Autodesk Inventor part; units mm, degrees
ref_plane "YZ Plane" through (0, 0, 0) normal (1, 0, 0) x (0, 1, 0)
ref_plane "XZ Plane" through (0, 0, 0) normal (0, 1, 0) x (-1, 0, 0)
ref_plane "XY Plane" through (0, 0, 0) normal (0, 0, 1) x (1, 0, 0)
sketch "Skizze1" plane through (0, 0, 0) normal (0, 0, 1) x (1, 0, 0)
  line L0 (13.8, 20) -> (-13.8, 20)
  line L1 (-13.8, 20) -> (-13.8, -20)
  line L2 (-13.8, -20) -> (13.8, -20)
  line L3 (13.8, 20) -> (-13.8, -20) construction
  line L4 (-13.8, 20) -> (13.8, -20) construction
  line L5 (13.8, 20) -> (13.8, 6.65) construction
  line L6 (13.8, 6.65) -> (10.7, 6.65)
  line L7 (-13.8, 0) -> (-0.95, 0) construction
  arc A0 (4.1513, 4.266) -> (4.1513, -4.266) centre (-0.95, 0) ccw
  line L8 (13.8, 6.65) -> (13.8, -6.65) construction
  line L9 (13.8, -6.65) -> (10.7, -6.65)
  line L10 (13.8, -20) -> (13.8, -6.65)
  line L11 (13.8, 6.65) -> (13.8, 20)
  line L12 (10.7, 6.65) -> (4.1513, 4.266)
  line L13 (10.7, -6.65) -> (4.1513, -4.266)
  point P0 (0, 0)
  dimension "d0" = 27.6
  dimension "d1" = 40
  dimension "d2" = 13.35
  dimension "d3" = 3.1
  dimension "d4" = 12.85
  dimension "d5" = 13.3
  dimension "d7" = 13.3
  dimension "d8" = 3.1
  dimension "d24" = 6.5487
  dimension "d25" = 6.5487
extrude "Extrusion1" add sketch "Skizze1" along normal blind 39
sketch "Skizze2" plane through (-13.8, -20, 0) normal (-1, 0, 0) x (0, 0, 1)
  line L0 (0, 40) -> (39, 40) construction
  line L1 (0, 0) -> (39, 0) construction
  line L2 (0, 40) -> (39, 0) construction
  line L3 (39, 40) -> (0, 0) construction
  line L4 (6.5, 6) -> (32.5, 6) construction
  line L5 (32.5, 6) -> (32.5, 34) construction
  line L6 (32.5, 34) -> (6.5, 34) construction
  line L7 (6.5, 34) -> (6.5, 6) construction
  line L8 (6.5, 6) -> (32.5, 34) construction
  line L9 (32.5, 6) -> (6.5, 34) construction
  point P0 (0, 20)
  point P1 (19.5, 20)
  dimension "d12" = 26
  dimension "d13" = 28
hole "Bohrung1" at (-13.8, 14, 6.5) at (-13.8, 14, 32.5) at (-13.8, -14, 32.5) at (-13.8, -14, 6.5) direction (1, 0, 0) diameter 3.242 depth 11.8 tip angle 118
chamfer "Fase1" distance 0.5 angle 45 26 edges at (13.8, 13.325, 39) (13.8, 13.325, 0) (13.8, -13.325, 0) (13.8, -13.325, 39) (13.8, -20, 19.5) (0, -20, 39) (-13.8, 0, 39) (0, 20, 39) (-13.8, 20, 19.5) (0, 20, 0) (13.8, 6.65, 19.5) (13.8, -6.65, 19.5) (-7.6, 0, 39) (7.4257, -5.458, 39) (12.25, -6.65, 39) (7.4257, 5.458, 39) (12.25, 6.65, 39) (-7.6, 0, 0) (7.4257, -5.458, 0) (12.25, -6.65, 0) (12.25, 6.65, 0) (7.4257, 5.458, 0) (0, -20, 0) (-13.8, -20, 19.5) (-13.8, 0, 0) (13.8, 20, 19.5)
chamfer_without_effect "Fase2"
properties part number "Führungswagen" material "Aluminium 6061"
CAD build for the part. Positions are in the model's coordinates, mm. A direction names the side the tool comes from. Coordinates: 2 decimals unless noted, no trailing zeros. Loops run counter-clockwise (first coordinate to the right, second up) from the corner with the lowest first, then second, coordinate; pieces in that order, holes last. Notation, with made-up numbers: (52.5, 4) - (99.5, 4) arc R32 ccw to (99.5, 37) - close; hole circle Ø9 at (53, 47.5). An arc over 180 degrees is marked (long way). Use one line per item in the form item = value. Start each with the question number.
1) Two-plate mould, pull along Z, no slides. Class faces 1 (the face through (-9, 0, 0)), 2 (the face through (13.8, -13, 19)), 3 (the face through (-7.817, 14.621, 33.997)): +Z half, -Z half, draft (parallel to the pull), parting line (faces both ways), or undercut.
2) Drill centre lines: L1, parallel to Z at x = -7.75, y = 14; L2, parallel to Y at x = -8, z = 32.5; L3, parallel to Y at x = -5.5, z = 32.5. Where is each one in solid material? Low to high. Write a range as from..to.
3) Band-saw the part on B-B (z = 19.5). Give the cut face in (x, y), and give its area (3 significant figures).
4) Band-saw the part on C-C (x = 11.25). Give the cut face in (y, z).
5) Flat gauge pins, fed straight in: pin 1 (2.5 mm diameter, centred on y = 14, z = 6.5, fed in from -X); pin 2 (3 mm diameter, centred on y = -14, z = 6.5, fed in from -X). Where does each tip first touch, or does it go through?
6) Tool access for faces 4 (the face through (7.471, -5.475, 19.234)), 5 (the face through (-7.817, 12.393, 6.289)), 6 (the face through (7.429, 5.722, 0.254)): list every direction of +Z, -Z, +X, -X, +Y, -Y with a clear straight run to the whole face (end or side of a thin tool).
7) Band-saw the part on A-A (x = -9). Give the cut face in (y, z).
8) Band-saw the part on D-D (y = 0). Give the cut face in (x, z), and give its area (3 significant figures).
Check values:
q1.face_1 = -Z half
q1.face_2 = draft
q1.face_3 = undercut
q2.L1 = 0..4.88, 8.12..30.88, 34.12..39
q2.L2 = -20..-15.62, -12.38..12.38, 15.62..20
q2.L3 = -20..-15.62, -12.38..-4.85, 4.85..12.38, 15.62..20
q3.outline = (-13.8, -19.5) - (-13.3, -20) - (13.3, -20) - (13.8, -19.5) - (13.8, -7.15) - (13.3, -6.65) - (10.7, -6.65) - (4.15, -4.27) arc R6.65 cw (long way) to (4.15, 4.27) - (10.7, 6.65) - (13.3, 6.65) - (13.8, 7.15) - (13.8, 19.5) - (13.3, 20) - (-13.3, 20) - (-13.8, 19.5) - close
q3.area = 861 mm2
q4.outline = (-20, 0.5) - (-19.5, 0) - (-7.15, 0) - (-6.65, 0.5) - (-6.65, 38.5) - (-7.15, 39) - (-19.5, 39) - (-20, 38.5) - close; (6.65, 0.5) - (7.15, 0) - (19.5, 0) - (20, 0.5) - (20, 38.5) - (19.5, 39) - (7.15, 39) - (6.65, 38.5) - close
q5.pin_1 = -1.78
q5.pin_2 = -1.93
q6.face_4 = +Z, -Z, +X
q6.face_5 = -X
q6.face_6 = -Z, +X
q7.outline = (-20, 0.5) - (-19.5, 0) - (19.5, 0) - (20, 0.5) - (20, 38.5) - (19.5, 39) - (-19.5, 39) - (-20, 38.5) - close; hole circle Ø3.24 at (-14, 6.5); hole circle Ø3.24 at (-14, 32.5); hole circle Ø3.24 at (14, 6.5); hole circle Ø3.24 at (14, 32.5)
q8.outline = (-13.8, 0.5) - (-13.3, 0) - (-8.1, 0) - (-7.6, 0.5) - (-7.6, 38.5) - (-8.1, 39) - (-13.3, 39) - (-13.8, 38.5) - close
q8.area = 241 mm2
